Model file for the job. Use its own axes, mm. A direction names the side the tool comes from. Round coordinates to 2 decimals unless told otherwise and drop trailing zeros. Loops run counter-clockwise (first coordinate to the right, second up) from the corner with the lowest first, then second, coordinate; pieces in that order, holes last. Notation, with made-up numbers: M 17.5,-20 L 26.5,-20 A11 cw 26.5,-1 Z; hole C -12.75,27 d3. An arc over 180 degrees is marked long. Use a Markdown table: item, result. Add a question column.
Q1. Probe line 1 (Y direction, x = -25.4, z = 23.5); line 2 (Y direction, x = -6, z = 8); line 3 (Z direction, x = -4, y = -1.5). List the from-to ranges inside material, lowest first. Write a range as from..to.
Q2. Pin check, flat tips, straight feed: pin 1 (8 mm diameter, centred on x = -13.5, z = 9.5, fed in from +Y); pin 2 (6 mm diameter, centred on y = -8, z = 7.5, fed in from -X); pin 3 (6 mm diameter, centred on y = -4.5, z = 13, fed in from -X); pin 4 (10 mm diameter, centred on x = 5, z = 4.5, fed in from -Y). Stop position of each tip, or through.
Q3. Mould opens along X. For faces 5 (the face through (-13.55, 3.33, 25.36)), 6 (the face through (-23, 8, 17.3)), 7 (the face through (0, 0, 19.05)), 8 (the face through (-15.736, -0.525, 15.773)) say: +X half, -X half, draft (parallel to the pull), parting line (faces both ways), or undercut.
Q4. Tool access for faces 1 (the face through (-7.559, 5.796, 9)), 2 (the face through (-14.288, -1, 6)), 3 (the face through (-12.41, -7.2, 6.59)), 4 (the face through (-30.162, 6, 21)): list every direction of +Z, -Z, +X, -X, +Y, -Y with a clear straight run to the whole face (end or side of a thin tool).
Q5. Cut at B-B (x = -25.4). Give the cut face in (y, z), plus the area to 3 significant figures.
Autodesk Inventor part; units mm, degrees
ref_plane "Work Plane1" through (0, 0, 19.05) normal (0, 0, -1) x (-1, 0, 0)
ref_plane "YZ Plane" through (0, 0, 0) normal (1, 0, 0) x (0, 1, 0)
ref_plane "XZ Plane" through (0, 0, 0) normal (0, 1, 0) x (-1, 0, 0)
sketch "Sketch1" plane through (0, 0, 0) normal (0, 0, 1) x (1, 0, 0)
  arc A0 (-3.9687, -12.064) -> (2.2782, 12.494) centre (0, 0) ccw
  circle A1 centre (-25.4, 0) radius 2.2479
  circle A2 centre (-25.4, 12.7) radius 2.2479
  line L0 (-25.4, 0) -> (-25.4, 12.7) construction
  line L1 (0, 0) -> (-25.4, 0) construction
  arc A3 (-24.5457, 17.3852) -> (-30.1625, 12.7) centre (-25.4, 12.7) ccw
  arc A4 (-30.1625, 0) -> (-26.8883, -4.524) centre (-25.4, 0) ccw
  line L2 (-26.8883, -4.524) -> (-3.9687, -12.064)
  line L3 (2.2782, 12.494) -> (-24.5457, 17.3852)
  line L4 (-30.1625, 12.7) -> (-30.1625, 0)
  circle A5 centre (0, 0) radius 9.525
  dimension "d0" = 25.4
  dimension "d1" = 12.7
  dimension "d2" = 4.4958
  dimension "d3" = 25.4
  dimension "d8" = 9.525
  dimension "d9" = 9.525
  dimension "d10" = 19.05
extrude "Extrusion1" add sketch "Sketch1" along normal blind 25.4
sketch "Sketch2" plane through (0, 0, 0) normal (0, 1, 0) x (-1, 0, 0)
  line L0 (-25.3065, 18.9574) -> (19.1186, 26.3269)
  line L1 (19.1186, 26.3269) -> (-25.6271, 26.3269)
  line L2 (-25.6271, 26.3269) -> (-25.3065, 18.9574)
  point P0 (0, 0)
extrude "Extrusion2" cut sketch "Sketch2" along normal through all both and the other way through all
fillet "Fillet1" radius 12.7 1 edges at (-13.531, 3.2293, 25.4)
ref_plane "Work Plane1" through (0, 0, 19.05) normal (0, 0, -1) x (-1, 0, 0)
sketch "Sketch4" plane through (-30.1625, 0, 0) normal (-1, 0, 0) x (0, 0, 1)
  line L0 (17.3005, 18.8893) -> (-1.1849, 18.8893)
  line L1 (-1.1849, 18.8893) -> (-1.1849, -14.6789)
  line L2 (-1.1849, -14.6789) -> (17.3005, -14.6789)
  line L3 (17.3005, -14.6789) -> (17.3005, 18.8893)
  point P0 (0, 0)
extrude "Extrusion4" cut sketch "Sketch4" against normal blind 15.875
fillet "Fillet2" radius 12.7 1 edges at (-14.2875, 15.5147, 8.6503)
fillet "Fillet3" radius 10.16 1 edges at (-14.2875, -8.6693, 8.6503)
fillet "Fillet4" radius 5.08 3 edges at (-12.358, -7.2729, 17.3005) (-9.7225, 10.042, 17.3005) (-14.2875, -0.5133, 17.3005)
sketch "Sketch6" plane through (0, 0, 19.05) normal (0, 0, -1) x (-1, 0, 0)
  circle A0 centre (0, 0) radius 9.525
  arc A1 (7.3025, -10.9672) -> (14.2875, -1.3161) centre (4.1275, -1.3161) ccw
  line L0 (14.2875, -1.3161) -> (14.2875, 0.2895)
  arc A2 (14.2875, 0.2895) -> (-0.6907, 12.7835) centre (1.5875, 0.2895) ccw
  line L1 (-2.2782, 12.494) -> (-0.6907, 12.7835)
  arc A3 (-2.2782, 12.494) -> (3.9687, -12.064) centre (0, 0) ccw
  line L2 (7.3025, -10.9672) -> (3.9687, -12.064)
extrude "Extrusion6" add sketch "Sketch6" against normal up to surface contours A0 surface through (25.3065, 0, 18.9574) normal (-0.1636509, 0, -0.9865183)
chamfer "Chamfer1" distance 0.7937 angle 45 1 edges at (-9.525, 0, 19.05)
chamfer "Chamfer2" distance 0.7937 angle 45 6 edges at (-9.7225, 10.042, 0) (-14.2875, -0.5133, 0) (-12.358, -7.2729, 0) (-5.6356, -11.5156, 0) (12.308, -3.1309, 0) (1.4845, 12.6387, 0)
properties part number "thing" material "white pla"
Checked values:
| question | item | result |
|---|---|---|
| 1 | line 1 | y = -5.01..-2.25, 2.25..10.45, 14.95..17.46 |
| 1 | line 2 | y = -11.4..-7.4, 7.4..12.2 |
| 1 | line 3 | z = 19.05..23.82 |
| 2 | pin 1 | stops at y = 10.22 |
| 2 | pin 2 | stops at x = -13.6 |
| 2 | pin 3 | stops at x = -15.62 |
| 2 | pin 4 | stops at y = -12.7 |
| 3 | face 5 | +X half |
| 3 | face 6 | draft |
| 3 | face 7 | undercut |
| 3 | face 8 | -X half |
| 4 | face 1 | -Z |
| 4 | face 2 | -Z, -X, +Y, -Y |
| 4 | face 3 | -Z, -X, -Y |
| 4 | face 4 | +Z, -Z, -X, +Y, -Y |
| 5 | outline | M -5.01,17.3 L -2.25,17.3 L -2.25,25.4 L -5.01,25.4 Z; M 2.25,17.3 L 10.45,17.3 L 10.45,25.4 L 2.25,25.4 Z; M 14.95,17.3 L 17.46,17.3 L 17.46,25.4 L 14.95,25.4 Z |
| 5 | area | 109 mm^2 |
